```python
from build123d import *

# Parameters (mm, degrees)
F2_W          = 3
F2_H          = 6.5
F3_DEPTH      = 25
F3_DEPTH_BACK = 25
F4_W          = 2.25
F4_H          = 6.5
F5_DEPTH      = 25
F5_DEPTH_BACK = 25
F6_R          = 1.5
F8_W          = 4
F8_H          = 2
F9_DEPTH      = 1
F10_SIZE2     = 1.99999
F10_SIZE      = 0.99999


# Not quite as in the source:
# - a fillet or chamfer is up to 0.001 mm smaller than in the source, because OpenCascade refuses the exact size


with BuildPart() as f1:
    # F0 (on Front) → F1 (revolve)
    with BuildSketch(Plane.XZ):
        Polygon((0, 2), (0, 0), (13.5, 0), (17, 3.5), (17, 13.5), (15, 13.5), (15, 4.3284271247), (12.6715728753, 2), align=None)
    revolve(axis=Axis((0, 0, 1), (0, 0, -1)))

    # F2 (on Right) → F3 (cut, two sides)
    with BuildSketch(Plane.YZ) as f3_sk:
        with Locations((0, 11.75)):
            Rectangle(F2_W, F2_H)
    extrude(amount=F3_DEPTH, mode=Mode.SUBTRACT)
    extrude(f3_sk.sketch, amount=-F3_DEPTH_BACK, mode=Mode.SUBTRACT)

    # F4 (on Front) → F5 (cut, two sides)
    with BuildSketch(Plane.XZ) as f5_sk:
        with Locations((-3.125, 11.75)):
            Rectangle(F4_W, F4_H)
        with Locations((3.125, 11.75)):
            Rectangle(F4_W, F4_H)
    extrude(amount=F5_DEPTH, mode=Mode.SUBTRACT)
    extrude(f5_sk.sketch, amount=-F5_DEPTH_BACK, mode=Mode.SUBTRACT)

    # F6
    f6_edges = [f1.edges().sort_by_distance(p)[0] for p in [
        (-12.671573, 0, 2),
        (-15, 0, 4.328427),
        (-17, 0, 3.5),
        (-13.5, 0, 0),
    ]]
    fillet(f6_edges, radius=F6_R)

    # F8 (on offset) → F9 (join)
    with BuildSketch(Plane.XZ.offset(16.88)):
        with Locations((0, 12.5)):
            Rectangle(F8_W, F8_H)
    extrude(amount=F9_DEPTH)

    # F10 (size 1 and 2 in the source; OpenCascade refuses exactly that, so slightly less here)
    f10_edges = [f1.edges().sort_by_distance(p)[0] for p in [
        (0, -17.88, 13.5),
    ]]
    f10_side = f1.faces().sort_by_distance((0, -16.417446, 13.5))[0]
    chamfer(f10_edges, length=F10_SIZE, length2=F10_SIZE2, reference=f10_side)

    # F11: F1 across plane


with BuildPart() as f1_1:
    add(f1.part)
    add(f1.part.mirror(Plane.XZ))


solid = f1_1.part
```
Build history of the part. All positions in model axes, mm. A direction names the side the tool comes from. Give positions to 0.01 mm unless a question says otherwise; leave off trailing zeros. Loops run counter-clockwise (first coordinate to the right, second up) from the corner with the lowest first, then second, coordinate; pieces in that order, holes last. Notation, with made-up numbers: (-32.5, 0) - (-0.5, 0) arc R18 cw to (-0.5, 9) - close; hole circle Ø5 at (53.25, -14.5). An arc over 180 degrees is marked (long way). Use a Markdown table: item, result.
(1) Band-saw the part on B-B (z = 6.25). Give the cut face in (x, y), and give its area (3 significant figures).
Taken from the geometry:
| item | result |
|---|---|
| outline | circle Ø34 at (0, 0); hole circle Ø30 at (0, 0) |
| area | 201 mm2 |
(2) Which spindle directions (+Z, -Z, +X, -X, +Y, -Y) get a long thin tool onto all of the face, cutting with end or side? Do faces 4 (the face through (-16, -1.5, 11)), 5 (the face through (-4.25, -15, 11)), 6 (the face through (0, 0, 0)), 7 (the face through (14.307, -4.506, 9.165)), 8 (the face through (-12, 9.5, 13.5)). Say none if no direction does.
Taken from the geometry:
| item | result |
|---|---|
| face 4 | +Z, +X, -X |
| face 5 | +Z, +Y, -Y |
| face 6 | -Z, +X, -X, +Y, -Y |
| face 7 | +Z |
| face 8 | +Z, +X, -X, +Y, -Y |
(3) Pull direction X, two halves, no side cores. Call faces 1 (the face through (13.45, -4.24, 0.6)), 2 (the face through (12, -10, 13.5)), 3 (the face through (0, 0, 2)): +X half, -X half, draft (parallel to the pull), parting line (faces both ways), or undercut.
Taken from the geometry:
| item | result |
|---|---|
| face 1 | parting line |
| face 2 | draft |
| face 3 | undercut |
(4) Band-saw the part on A-A (z = 10.75). Give the cut face in (x, y), and give its area (3 significant figures).
Taken from the geometry:
| item | result |
|---|---|
| outline | (-16.93, -1.5) arc R17 ccw to (-4.25, -16.46) - (-4.25, -14.39) arc R15 cw to (-14.92, -1.5) - close; (-16.93, 1.5) - (-14.92, 1.5) arc R15 cw to (-4.25, 14.39) - (-4.25, 16.46) arc R17 ccw to start; (-2, -16.88) arc R17 ccw to (2, -16.88) - (2, -14.87) arc R15 cw to (-2, -14.87) - close; (-2, 14.87) arc R15 cw to (2, 14.87) - (2, 16.88) arc R17 ccw to (-2, 16.88) - close; (4.25, -16.46) arc R17 ccw to (16.93, -1.5) - (14.92, -1.5) arc R15 cw to (4.25, -14.39) - close; (4.25, 14.39) arc R15 cw to (14.92, 1.5) - (16.93, 1.5) arc R17 ccw to (4.25, 16.46) - close |
| area | 171 mm2 |
(5) Wall check: line 1 along Y through (x, z) = (0, 11); line 2 along Z through (x, y) = (4, 3). Give the ranges that are in metal, low to high.
Taken from the geometry:
| item | result |
|---|---|
| line 1 | -17 to -15, 15 to 17 |
| line 2 | 0 to 2 |
(6) Drop flat-ended pins along their axis: pin 1 Ø1.6 at (x, z) = (-15.5, 10) entering from +Y; pin 2 Ø8 at (x, z) = (-11, 10.5) entering from -Y; pin 3 Ø3.5 at (y, z) = (16.5, 11.5) entering from -X. Give the stop position or say it passes through.
Taken from the geometry:
| item | result |
|---|---|
| pin 1 | y = 8.54 |
| pin 2 | y = -15.49 |
| pin 3 | x = -8.45 |
